Could you check a few things on this model? Use its own coordinates, in mm. Coordinates: 2 decimals unless noted, no trailing zeros. Order: outer loops, then holes, each group sorted by start corner. A loop starts at its lowest first (then second) coordinate and runs counter-clockwise, first axis right, second up. Notation, with made-up numbers: (13, 47.5) -> (22, 47.5) arc R26 ccw to (22, 68.5) -> close; hole circle Ø10 at (35, -21). An arc over 180 degrees is marked (long way). Use a Markdown table: item, result. Add a question column.
1) If I drill on L1, parallel to Z at x = -27.5, y = 0.3; L2, parallel to X at y = 0.7, z = 95; L3, parallel to X at y = 0.6, z = 99, over which ranges is the centre line in solid material (lowest first)? Write a range as [from, to].
2) If we section it at B-B (x = 41): Write out the boundary of the cut face in (y, z).
3) If we section it at C-C (z = 87): Write out the boundary of the cut face in (x, y).
4) If we section it at A-A (y = 3.2): Write out the boundary of the cut face in (x, z).
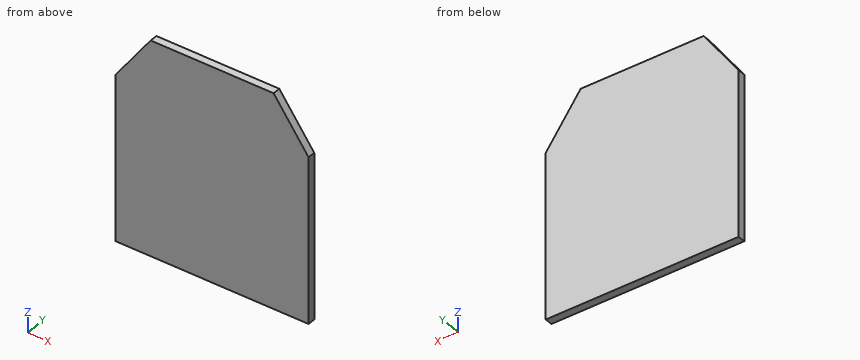
```python
from build123d import *

# Parameters (mm, degrees)
SKETCH1_W           = 100
SKETCH1_H           = 85
BOSS_EXTRUDE1_DEPTH = 4


with BuildPart() as part:
    # Sketch1 → Boss-Extrude1 (new body)
    with BuildSketch(Plane(origin=(0, 0, 0), x_dir=(1, 0, 0), z_dir=(0, 1, 0))):
        Polygon((-45.143769968, -85), (54.856230032, -85), (36.741214058, -110), (-27.028753994, -110), align=None)
        with Locations((4.856230032, -42.5)):
            Rectangle(SKETCH1_W, SKETCH1_H)
    extrude(amount=BOSS_EXTRUDE1_DEPTH)


solid = part.part
```
Answer sheet:
| question | item | result |
|---|---|---|
| 1 | L1 | [0, 109.35] |
| 1 | L2 | [-37.9, 47.61] |
| 1 | L3 | [-35, 44.71] |
| 2 | outline | (0, 0) -> (4, 0) -> (4, 104.12) -> (0, 104.12) -> close |
| 3 | outline | (-43.69, 0) -> (53.41, 0) -> (53.41, 4) -> (-43.69, 4) -> close |
| 4 | outline | (-45.14, 0) -> (54.86, 0) -> (54.86, 85) -> (36.74, 110) -> (-27.03, 110) -> (-45.14, 85) -> close |
